Verification items for the finished model (mm, model axes). Face numbers are marked on the shaded views. A direction names the side the tool comes from. Give positions to 0.01 mm unless a question says otherwise; leave off trailing zeros. Order: outer loops, then holes, each group sorted by start corner. A loop starts at its lowest first (then second) coordinate and runs counter-clockwise, first axis right, second up. Notation, with made-up numbers: M 74,-29.5 L 99,-29.5 A21 ccw 99,-0.5 Z; hole C 87,83.5 d6. An arc over 180 degrees is marked long. Answer as a JSON object with one key per item and string values.
```python
from build123d import *

# Parameters (mm, degrees)
F0_R     = 7.5
F1_DEPTH = 16
F3_DEPTH = 16
F4_COUNT = 10
F5_R     = 7.5
F6_DEPTH = 3
F8_DEPTH = 3


with BuildPart() as f1:
    # F0 (on Top) → F1 (new body)
    with BuildSketch(Plane.XY):
        Circle(F0_R)
        with BuildLine():
            ThreePointArc((1.6278820596, 2.4), (0, -2.9), (-1.6278820596, 2.4))
            Line((-1.6278820596, 2.4), (1.6278820596, 2.4))
        make_face(mode=Mode.SUBTRACT)
    extrude(amount=F1_DEPTH)

    # F2 (on face) → F3 (cut, through all)
    with BuildSketch(Plane.XY.offset(16)):
        with BuildLine():
            ThreePointArc((0.45, 4.477443467), (0.833787098, 6.0733536603), (2, 7.2284161474))
            ThreePointArc((2, 7.2284161474), (0, 7.5), (-2, 7.2284161474))
            ThreePointArc((-2, 7.2284161474), (-0.833787098, 6.0733536603), (-0.45, 4.477443467))
            ThreePointArc((-0.45, 4.477443467), (0, 4.5), (0.45, 4.477443467))
        make_face()
    f3 = extrude(amount=-F3_DEPTH, mode=Mode.SUBTRACT)

    # F4: F3 ×10 about axis
    f4_axis = Axis((0, 0, 0), (0, 0, -1))
    for i in range(1, F4_COUNT):
        add(f3.rotate(f4_axis, i * 360 / F4_COUNT), mode=Mode.SUBTRACT)

    # F5 (on Top) → F6 (join)
    with BuildSketch(Plane.XY):
        Circle(F5_R)
    extrude(amount=F6_DEPTH)

    # F7 (on face) → F8 (cut, through all)
    with BuildSketch(Plane.XY.offset(3)):
        with BuildLine():
            Line((1.6278820596, 2.4), (-1.6278820596, 2.4))
            ThreePointArc((-1.6278820596, 2.4), (0, -2.9), (1.6278820596, 2.4))
        make_face()
    extrude(amount=-F8_DEPTH, mode=Mode.SUBTRACT)


solid = f1.part
```
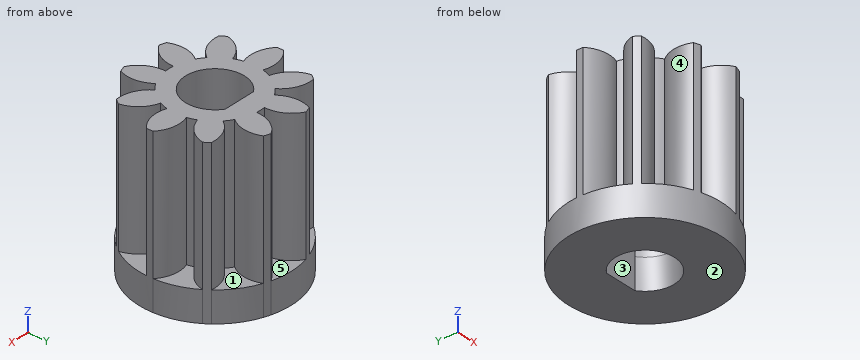
Q1. Gauge pin test, flat ends, axial feed: pin 1 Ø1.1 at (x, y) = (4, -5) entering from +Z; pin 2 Ø4 at (x, z) = (-2, 6) entering from -Y; pin 3 Ø2 at (x, z) = (-6, 7.5) entering from +Y. Record the tip position at first contact, or that the pin passes through.
Resolved:
{"pin 1": "stops at z = 3", "pin 2": "stops at y = -7.23", "pin 3": "stops at y = 4.7"}
Q2. Release check for a two-part mould opening along Y. For the marked faces 3, 4 and 5 record: +Y half, -Y half, draft (parallel to the pull), parting line (faces both ways), or undercut.
Resolved:
{"face 3": "undercut", "face 4": "undercut", "face 5": "draft"}
Q3. Section check C-C on x = -6.5. Record the cut outline in (y, z), then the cut area to 3 significant figures.
Resolved:
{"outline": "M -3.74,0 L 3.74,0 L 3.74,3 L 0.95,3 L 0.95,16 L -0.95,16 L -0.95,3 L -3.74,3 Z", "area": "47.1 mm²"}
Q4. Tool access check on the marked faces 1 and 2. Record the directions out of +Z, -Z, +X, -X, +Y, -Y that give a thin tool (end or side, any length) a straight path to the whole face; none if there is none.
Resolved:
{"face 1": "+Z", "face 2": "-Z, +X, -X, +Y, -Y"}
Q5. Section check B-B on x = 0. Record the cut outline in (y, z), then the cut area to 3 significant figures.
Resolved:
{"outline": "M -7.5,0 L -2.9,0 L -2.9,16 L -4.5,16 L -4.5,3 L -7.5,3 Z; M 2.4,0 L 7.5,0 L 7.5,3 L 4.5,3 L 4.5,16 L 2.4,16 Z", "area": "77.2 mm²"}
Q6. Material ranges on L1, parallel to X at y = 3.5, z = 7.25; L2, parallel to Y at x = -4.5, z = 8.5; L3, parallel to X at y = 4, z = 11, recorded low to high.
Resolved:
{"L1": "x = -6.06 to -3.1, -2.83 to 2.83, 3.1 to 6.06", "L2": "y = -4.53 to -1.95, -0.99 to 0.99, 1.95 to 4.53", "L3": "x = -6.23 to -3.57, -2.35 to 2.35, 3.57 to 6.23"}
Q7. Section check A-A on y = 0. Record the cut outline in (x, z), then the cut area to 3 significant figures.
Resolved:
{"outline": "M -7.5,0 L -2.9,0 L -2.9,16 L -7.5,16 Z; M 2.9,0 L 7.5,0 L 7.5,16 L 2.9,16 Z", "area": "147 mm²"}
Q8. Section check D-D on y = -5.5. Record the cut outline in (x, z).
Resolved:
{"outline": "M -5.1,0 L 5.1,0 L 5.1,3 L 2.9,3 L 2.9,16 L 0.59,16 L 0.59,3 L -0.59,3 L -0.59,16 L -2.9,16 L -2.9,3 L -5.1,3 Z"}
